from build123d import *

# Parameters (mm, degrees)
SZKIC1_W = 3
SZKIC1_H = 15


with BuildPart() as part:
    # Szkic1 → Obrót1 (revolve)
    with BuildSketch(Plane.XY, mode=Mode.PRIVATE) as obr_t1_sk:
        Polygon((-65, 0), (-62, 0), (-62, 20), (-60, 20), (-58, 30), (-58, 60), (-61, 60), (-61, 90), (-64, 90), (-65, 90), (-65, 20), align=None)
        with Locations((-62.5, 97.5)):
            Rectangle(SZKIC1_W, SZKIC1_H)
    revolve(obr_t1_sk.sketch.rotate(Axis((0, 0, 0), (0, 1, 0)), 270), axis=Axis((0, 0, 0), (0, 1, 0)))


solid = part.part
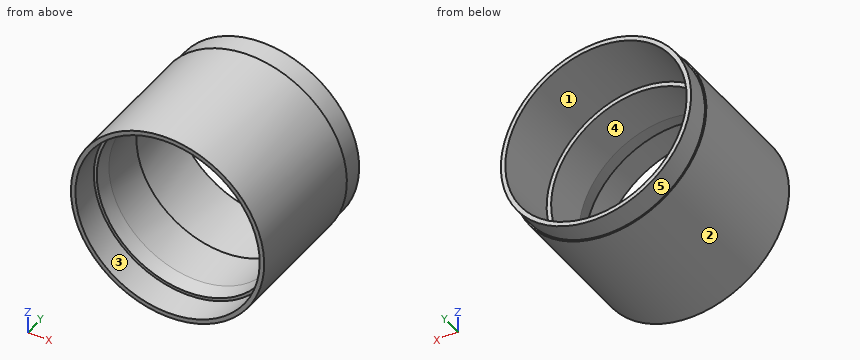
Check sheet for the modelled part. Datum: model origin and axes. Units: mm. Face numbers are marked on the shaded views. A direction names the side the tool comes from. Round coordinates to 2 decimals unless told otherwise and drop trailing zeros. Order: outer loops, then holes, each group sorted by start corner. A loop starts at its lowest first (then second) coordinate and runs counter-clockwise, first axis right, second up. Notation, with made-up numbers: M 6.5,14.5 L 35.5,14.5 A23 ccw 35.5,38.5 Z; hole C 64,41.25 d9. An arc over 180 degrees is marked long. One line per item, written item: value. Start each with the question number.
1. Scan lines: line 1 along X through (y, z) = (51.5, 0); line 2 along Z through (x, y) = (10, 46); line 3 along X through (y, z) = (15.5, 0). Record each from-to range of solid material in increasing order.
2. Section check D-D on y = 84. Enter the section's corners in (x, z).
3. Release check for a two-part mould opening along Z. For the marked faces 1, 2 and 3 record: released by +Z, released by -Z, zero draft, split by the parting line, or undercut.
4. Access from +Z, -Z, +X, -X, +Y, -Y to the whole of each face (thin tool, end or side, straight path). Record for the marked faces 4 and 5.
5. Gauge pin test, flat ends, axial feed: P1, Ø1.5, axis at x = -5, y = 91, coming from the -Z side; P2, Ø4, axis at x = 17.5, y = 69.5, coming from the +Z side; P3, Ø5, axis at x = -40.5, y = 74, coming from the +Z side. Record the tip position at first contact, or that the pin passes through.
6. Section check A-A on x = 0. Enter the section's corners in (y, z), and give its area (3 significant figures).
7. Section check B-B on z = 0. Enter the section's corners in (x, y).
8. Section check C-C on y = 96. Enter the section's corners in (x, z).
Results found:
1. line 1: -65 to -58, 58 to 65
1. line 2: -64.23 to -57.13, 57.13 to 64.23
1. line 3: -65 to -62, 62 to 65
2. outline: C 0,0 d130; hole C 0,0 d122
3. face 1: undercut
3. face 2: split by the parting line
3. face 3: undercut
4. face 4: +Y, -Y
4. face 5: +Y
5. P1: z = -63.86
5. P2: z = 63.12
5. P3: z = 52.74
6. outline: M 0,-65 L 90,-65 L 90,-64 L 105,-64 L 105,-61 L 60,-61 L 60,-58 L 30,-58 L 20,-60 L 20,-62 L 0,-62 Z; M 0,62 L 20,62 L 20,60 L 30,58 L 60,58 L 60,61 L 105,61 L 105,64 L 90,64 L 90,65 L 0,65 Z
6. area: 990 mm^2
7. outline: M -65,0 L -62,0 L -62,20 L -60,20 L -58,30 L -58,60 L -61,60 L -61,105 L -64,105 L -64,90 L -65,90 Z; M 58,30 L 60,20 L 62,20 L 62,0 L 65,0 L 65,90 L 64,90 L 64,105 L 61,105 L 61,60 L 58,60 Z
8. outline: C 0,0 d128; hole C 0,0 d122
